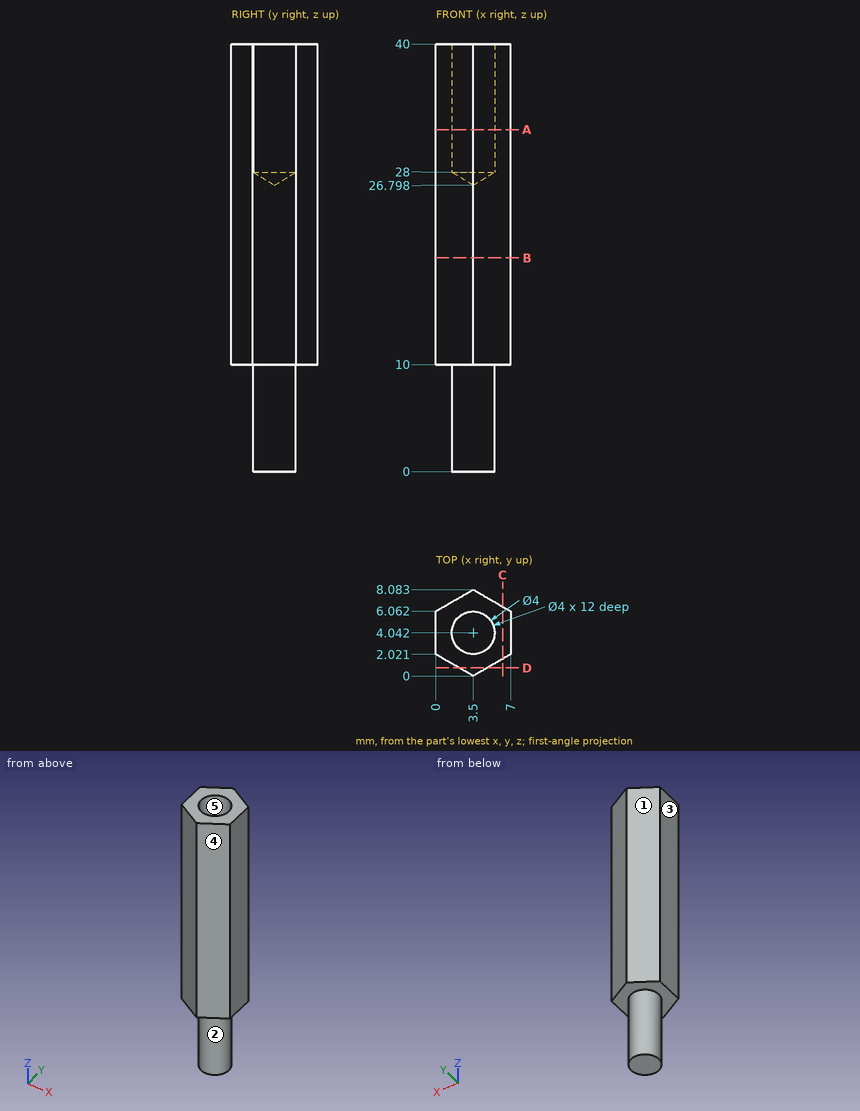
Can you work these out from the drawing? Everything is in mm from the part's minimum corner. A direction names the side the tool comes from. Coordinates: 2 decimals unless noted, no trailing zeros. Order: outer loops, then holes, each group sorted by start corner. A loop starts at its lowest first (then second) coordinate and runs counter-clockwise, first axis right, second up. Notation, with made-up numbers: (74.5, 47) -> (116.5, 47) arc R13 cw to (116.5, 66) -> close; hole circle Ø6 at (-11, 17.5). An arc over 180 degrees is marked (long way). Return JSON: item names as keys, results as strings.
1) If we section it at D-D on y = 0.75: List the corners of the cut face in (x, z) for me.
Conclusion:
{"outline": "(2.2, 10) -> (4.8, 10) -> (4.8, 40) -> (2.2, 40) -> close"}
2) If we section it at A-A on z = 32: List the corners of the cut face in (x, y) for me.
Conclusion:
{"outline": "(0, 2.02) -> (3.5, 0) -> (7, 2.02) -> (7, 6.06) -> (3.5, 8.08) -> (0, 6.06) -> close; hole circle Ø4 at (3.5, 4.04)"}
3) If I drill on probe 1 along Z at (x, y) = (4.25, 0.5); probe 2 along X at (y, z) = (4.5, 38); probe 3 along X at (y, z) = (4.25, 27) (1 decimal), over which ranges is the centre line in solid material (lowest first)?
Conclusion:
{"probe 1": "z = 10 to 40", "probe 2": "x = 0 to 1.55, 5.45 to 7", "probe 3": "x = 0 to 3.2, 3.8 to 7"}
4) Thinking about a two-plate mould opening in Y: for the marked faces 3, 4 and 5, which applies, +Y half, -Y half, draft (parallel to the pull), parting line (faces both ways), or undercut?
Conclusion:
{"face 3": "draft", "face 4": "-Y half", "face 5": "undercut"}
5) On a 3-axis mill with a long thin cutter (end or side, diameter ignored), from which of +Z, -Z, +X, -X, +Y, -Y can I reach the whole of each face in a straight line? I mean the marked faces 1 and 2. Say none if no direction works.
Conclusion:
{"face 1": "+Z, -Z, -X, +Y", "face 2": "-Z"}
6) If we section it at C-C on x = 6.25: List the corners of the cut face in (y, z) for me (1 decimal), plus the area to 3 significant figures.
Conclusion:
{"outline": "(1.6, 10) -> (6.5, 10) -> (6.5, 40) -> (1.6, 40) -> close", "area": "147 mm²"}
7) I'm going to push a flat-ended pin straight in: P1, Ø2, axis at x = 6, z = 34, coming from the +Y side. Where does the tip first touch, or does it pass through?
Conclusion:
{"P1": "stops at y = 7.22"}
8) If we section it at B-B on z = 20: List the corners of the cut face in (x, y) for me.
Conclusion:
{"outline": "(0, 2.02) -> (3.5, 0) -> (7, 2.02) -> (7, 6.06) -> (3.5, 8.08) -> (0, 6.06) -> close"}
